from build123d import *

# Parameters (mm, degrees)
F0_W          = 55
F0_H          = 70
F1_DEPTH      = 10
F2_W          = 99
F2_H          = 59
F3_DEPTH      = 5
F4_W          = 110
F4_H          = 70
F4_W_2        = 99
F4_H_2        = 59
F4_W_3        = 95
F4_H_3        = 55
F5_DEPTH      = 3
F6_W          = 110
F6_H          = 70
F6_W_2        = 99
F6_H_2        = 59
F7_DEPTH      = 10
F8_R          = 4
F9_R          = 3
F10_T1_DEPTH  = 59
F10_T3_DEPTH  = 99
F10_T9_DEPTH  = 106.5
F10_T13_DEPTH = 66.5
F10_T20_DEPTH = 66.5
F10_T24_DEPTH = 106.5
F10_T31_DEPTH = 106.5
F10_T35_DEPTH = 66.5
F10_T42_DEPTH = 106.5
F10_T46_DEPTH = 66.5


# Not quite as in the source:
# - a fillet or chamfer that OpenCascade refuses, or shapes differently, is made with other operations: its cross-section is extruded or revolved along the edge and cut away or added


with BuildPart() as f1:
    # F0 (on Front) → F1 (new body)
    with BuildSketch(Plane.XZ):
        with Locations((-27.5, 0)):
            Rectangle(F0_W, F0_H)
        with Locations((27.5, 0)):
            Rectangle(F0_W, F0_H)
    extrude(amount=F1_DEPTH)

    # F2 (on face) → F3 (cut)
    with BuildSketch(Plane.XZ.offset(10)):
        Rectangle(F2_W, F2_H)
    extrude(amount=-F3_DEPTH, mode=Mode.SUBTRACT)

    # F4 (on face) → F5 (join)
    with BuildSketch(Plane.XZ.offset(10)):
        Rectangle(F4_W, F4_H)
        Rectangle(F4_W_2, F4_H_2, mode=Mode.SUBTRACT)
        Rectangle(F4_W_2, F4_H_2)
        Rectangle(F4_W_3, F4_H_3, mode=Mode.SUBTRACT)
    extrude(amount=F5_DEPTH)

    # F6 (on face) → F7 (join)
    with BuildSketch(Plane.XZ.offset(13)):
        Rectangle(F6_W, F6_H)
        Rectangle(F6_W_2, F6_H_2, mode=Mode.SUBTRACT)
    extrude(amount=F7_DEPTH)

    # F8
    f8_edges = [f1.edges().sort_by_distance(p)[0] for p in [
        (0, 0, 35),
        (-55, 0, 0),
        (55, 0, 0),
        (0, 0, -35),
    ]]
    fillet(f8_edges, radius=F8_R)

    # F9
    f9_edges = [f1.edges().sort_by_distance(p)[0] for p in [
        (-55, -23, 0),
        (0, -23, 35),
        (0, -23, -35),
        (55, -23, 0),
    ]]
    fillet(f9_edges, radius=F9_R)

    # F10: fillet of radius 3 on 4 edges, made by hand

    # F10_s2 → F10_t1 (cut)
    with BuildSketch(Plane.XY.offset(-29.5)):
        with BuildLine():
            ThreePointArc((-52.5, -23), (-50.3786796564, -22.1213203436), (-49.5, -20))
            Line((-49.5, -20), (-49.5, -23))
            Line((-49.5, -23), (-52.5, -23))
        make_face()
        with BuildLine():
            ThreePointArc((52.5, -23), (50.3786796564, -22.1213203436), (49.5, -20))
            Line((49.5, -20), (49.5, -23))
            Line((49.5, -23), (52.5, -23))
        make_face()
    extrude(amount=F10_T1_DEPTH, mode=Mode.SUBTRACT)

    # F10_s4 → F10_t3 (cut)
    with BuildSketch(Plane.YZ.offset(-49.5)):
        with BuildLine():
            ThreePointArc((-23, 32.5), (-22.1213203436, 30.3786796564), (-20, 29.5))
            Line((-20, 29.5), (-23, 29.5))
            Line((-23, 29.5), (-23, 32.5))
        make_face()
        with BuildLine():
            ThreePointArc((-23, -32.5), (-22.1213203436, -30.3786796564), (-20, -29.5))
            Line((-20, -29.5), (-23, -29.5))
            Line((-23, -29.5), (-23, -32.5))
        make_face()
    extrude(amount=F10_T3_DEPTH, mode=Mode.SUBTRACT)


with BuildPart() as f10_tool7:
    # F10_s8 → F10_t9 (new body)
    with BuildSketch(Plane.YZ.offset(49.5)):
        with BuildLine():
            ThreePointArc((-23, -32.5), (-22.1213203436, -30.3786796564), (-20, -29.5))
            Line((-20, -29.5), (-23, -29.5))
            Line((-23, -29.5), (-23, -32.5))
        make_face()
    extrude(amount=-F10_T9_DEPTH)

    split(bisect_by=Plane.YZ.offset(-49.5), keep=Keep.BOTTOM)


with BuildPart() as f10_tool11:
    # F10_s12 → F10_t13 (new body)
    with BuildSketch(Plane.XY.offset(-37)):
        with BuildLine():
            ThreePointArc((-52.5, -23), (-50.3786796564, -22.1213203436), (-49.5, -20))
            Line((-49.5, -20), (-49.5, -23))
            Line((-49.5, -23), (-52.5, -23))
        make_face()
    extrude(amount=F10_T13_DEPTH)

    split(bisect_by=Plane.XY.offset(-29.5), keep=Keep.BOTTOM)


with BuildPart() as f10_tool7_1:
    add(f10_tool7.part)

    # F10_t15: intersect F10_tool11
    add(f10_tool11.part, mode=Mode.INTERSECT)


with BuildPart() as f1_1:
    add(f1.part)

    # F10_t5: cut F10_tool7
    add(f10_tool7_1.part, mode=Mode.SUBTRACT)


with BuildPart() as f10_tool18:
    # F10_s19 → F10_t20 (new body)
    with BuildSketch(Plane.XY.offset(-29.5)):
        with BuildLine():
            ThreePointArc((-52.5, -23), (-50.3786796564, -22.1213203436), (-49.5, -20))
            Line((-49.5, -20), (-49.5, -23))
            Line((-49.5, -23), (-52.5, -23))
        make_face()
    extrude(amount=F10_T20_DEPTH)

    split(bisect_by=Plane.XY.offset(29.5), keep=Keep.TOP)


with BuildPart() as f10_tool22:
    # F10_s23 → F10_t24 (new body)
    with BuildSketch(Plane.YZ.offset(-57)):
        with BuildLine():
            ThreePointArc((-23, 32.5), (-22.1213203436, 30.3786796564), (-20, 29.5))
            Line((-20, 29.5), (-23, 29.5))
            Line((-23, 29.5), (-23, 32.5))
        make_face()
    extrude(amount=F10_T24_DEPTH)

    split(bisect_by=Plane.YZ.offset(-49.5), keep=Keep.BOTTOM)


with BuildPart() as f10_tool18_1:
    add(f10_tool18.part)

    # F10_t26: intersect F10_tool22
    add(f10_tool22.part, mode=Mode.INTERSECT)


with BuildPart() as f1_2:
    add(f1_1.part)

    # F10_t16: cut F10_tool18
    add(f10_tool18_1.part, mode=Mode.SUBTRACT)


with BuildPart() as f10_tool29:
    # F10_s30 → F10_t31 (new body)
    with BuildSketch(Plane.YZ.offset(-49.5)):
        with BuildLine():
            ThreePointArc((-23, 32.5), (-22.1213203436, 30.3786796564), (-20, 29.5))
            Line((-20, 29.5), (-23, 29.5))
            Line((-23, 29.5), (-23, 32.5))
        make_face()
    extrude(amount=F10_T31_DEPTH)

    split(bisect_by=Plane.YZ.offset(49.5), keep=Keep.TOP)


with BuildPart() as f10_tool33:
    # F10_s34 → F10_t35 (new body)
    with BuildSketch(Plane.XY.offset(37)):
        with BuildLine():
            ThreePointArc((52.5, -23), (50.3786796564, -22.1213203436), (49.5, -20))
            Line((49.5, -20), (49.5, -23))
            Line((49.5, -23), (52.5, -23))
        make_face()
    extrude(amount=-F10_T35_DEPTH)

    split(bisect_by=Plane.XY.offset(29.5), keep=Keep.TOP)


with BuildPart() as f10_tool29_1:
    add(f10_tool29.part)

    # F10_t37: intersect F10_tool33
    add(f10_tool33.part, mode=Mode.INTERSECT)


with BuildPart() as f1_3:
    add(f1_2.part)

    # F10_t27: cut F10_tool29
    add(f10_tool29_1.part, mode=Mode.SUBTRACT)


with BuildPart() as f10_tool40:
    # F10_s41 → F10_t42 (new body)
    with BuildSketch(Plane.YZ.offset(57)):
        with BuildLine():
            ThreePointArc((-23, -32.5), (-22.1213203436, -30.3786796564), (-20, -29.5))
            Line((-20, -29.5), (-23, -29.5))
            Line((-23, -29.5), (-23, -32.5))
        make_face()
    extrude(amount=-F10_T42_DEPTH)

    split(bisect_by=Plane.YZ.offset(49.5), keep=Keep.TOP)


with BuildPart() as f10_tool44:
    # F10_s45 → F10_t46 (new body)
    with BuildSketch(Plane.XY.offset(29.5)):
        with BuildLine():
            ThreePointArc((52.5, -23), (50.3786796564, -22.1213203436), (49.5, -20))
            Line((49.5, -20), (49.5, -23))
            Line((49.5, -23), (52.5, -23))
        make_face()
    extrude(amount=-F10_T46_DEPTH)

    split(bisect_by=Plane.XY.offset(-29.5), keep=Keep.BOTTOM)


with BuildPart() as f10_tool40_1:
    add(f10_tool40.part)

    # F10_t48: intersect F10_tool44
    add(f10_tool44.part, mode=Mode.INTERSECT)


with BuildPart() as f1_4:
    add(f1_3.part)

    # F10_t38: cut F10_tool40
    add(f10_tool40_1.part, mode=Mode.SUBTRACT)


solid = f1_4.part
Input: part model. Units: mm. Frame: model coordinates. A direction names the side the tool comes from. Coordinates: 2 decimals unless noted, no trailing zeros. Write each loop counter-clockwise with the first axis right and the second up, starting at its lowest first coordinate (ties: lowest second). Pieces come first, ordered by that corner, then holes. Notation, with made-up numbers: M 62,-18 L 98,-18 A28 ccw 98,19 Z; hole C -34,71 d9. An arc over 180 degrees is marked long. Answer as a JSON object with one key per item and string values. Group by question number.
(1) Set-up query: faces 1 (the face through (-50.31, -22.05, -0.45)), 2 (the face through (-1, -12, -35)), 3 (the face through (-1, -8, -29.5)). Return all of +Z, -Z, +X, -X, +Y, -Y with unobstructed straight access to the full face (end or side cutting, diameter ignored); none if empty.
(2) Section C-C on z = 25.5. Output: boundary loops of the cut face in (x, y).
(3) Section A-A on y = -6.25. Output: boundary loops of the cut face in (x, z), plus the area to 3 significant figures.
(4) Section D-D on y = -21.5. Output: boundary loops of the cut face in (x, z), plus the area to 3 significant figures.
(5) Ray query, line 1 along Z through (x, y) = (24, -19.75); line 2 along X through (y, z) = (-18, 20.5); line 3 along Y through (x, z) = (14, -28). Return the intervals inside material, ascending. Write a range as [from, to].
(6) Mould query, pull axis Y, two halves, no side actions, for faces 4 (the face through (49.5, -8, 0)), 5 (the face through (0.77, -1.203, -33.859)), 6 (the face through (-47.5, -11, 0)). Classes: pulls with the +Y half, pulls with the -Y half, needs draft (parallel to the pull), parting line crosses it, or undercut.
(7) Section B-B on x = 4.5. Output: boundary loops of the cut face in (y, z).
(8) Contact query for a flat-ended pin moving along its axis: P1, Ø2, axis at x = 18.5, z = -18, coming from the -Y side. Output: stop coordinate, or through.
Result set:
{
 "1": {"face 1": "-Y", "face 2": "-Z, +X, -X, +Y, -Y", "face 3": "none"},
 "2": {"outline": "M -55,-20 A3 ccw -52.25,-22.99 A3 ccw -49.5,-20 L -49.5,-13 L -47.5,-13 L -47.5,-10 L -49.5,-10 L -49.5,-5 L 49.5,-5 L 49.5,-10 L 47.5,-10 L 47.5,-13 L 49.5,-13 L 49.5,-20 A3 ccw 52.25,-22.99 A3 ccw 55,-20 L 55,-4 A4 ccw 51,0 L -51,0 A4 ccw -55,-4 Z"},
 "3": {"outline": "M -55,-35 L 55,-35 L 55,35 L -55,35 Z; hole M -49.5,-29.5 L 49.5,-29.5 L 49.5,29.5 L -49.5,29.5 Z", "area": "1,860 mm2"},
 "4": {"outline": "M -54.6,-34.6 L 54.6,-34.6 L 54.6,34.6 L -54.6,34.6 Z; hole M -49.9,-29.9 L 49.9,-29.9 L 49.9,29.9 L -49.9,29.9 Z", "area": "1,590 mm2"},
 "5": {"line 1": "z = [-35, -29.5], [29.5, 35]", "line 2": "x = [-55, -49.5], [49.5, 55]", "line 3": "y = [-13, -10], [-5, 0]"},
 "6": {"face 4": "undercut", "face 5": "pulls with the +Y half", "face 6": "needs draft"},
 "7": {"outline": "M -22.99,-32.25 A3 ccw -20,-35 L -4,-35 A4 ccw 0,-31 L 0,31 A4 ccw -4,35 L -20,35 A3 ccw -22.99,32.25 A3 ccw -20,29.5 L -13,29.5 L -13,27.5 L -10,27.5 L -10,29.5 L -5,29.5 L -5,-29.5 L -10,-29.5 L -10,-27.5 L -13,-27.5 L -13,-29.5 L -20,-29.5 A3 ccw Z"},
 "8": {"P1": "stops at y = -5"}
}
